Part print with two shaded views. Sizes in mm from the minimum x, y, z corner. A direction names the side the tool comes from. Round coordinates to 2 decimals unless told otherwise and drop trailing zeros. Write each loop counter-clockwise with the first axis right and the second up, starting at its lowest first coordinate (ties: lowest second). Pieces come first, ordered by that corner, then holes.
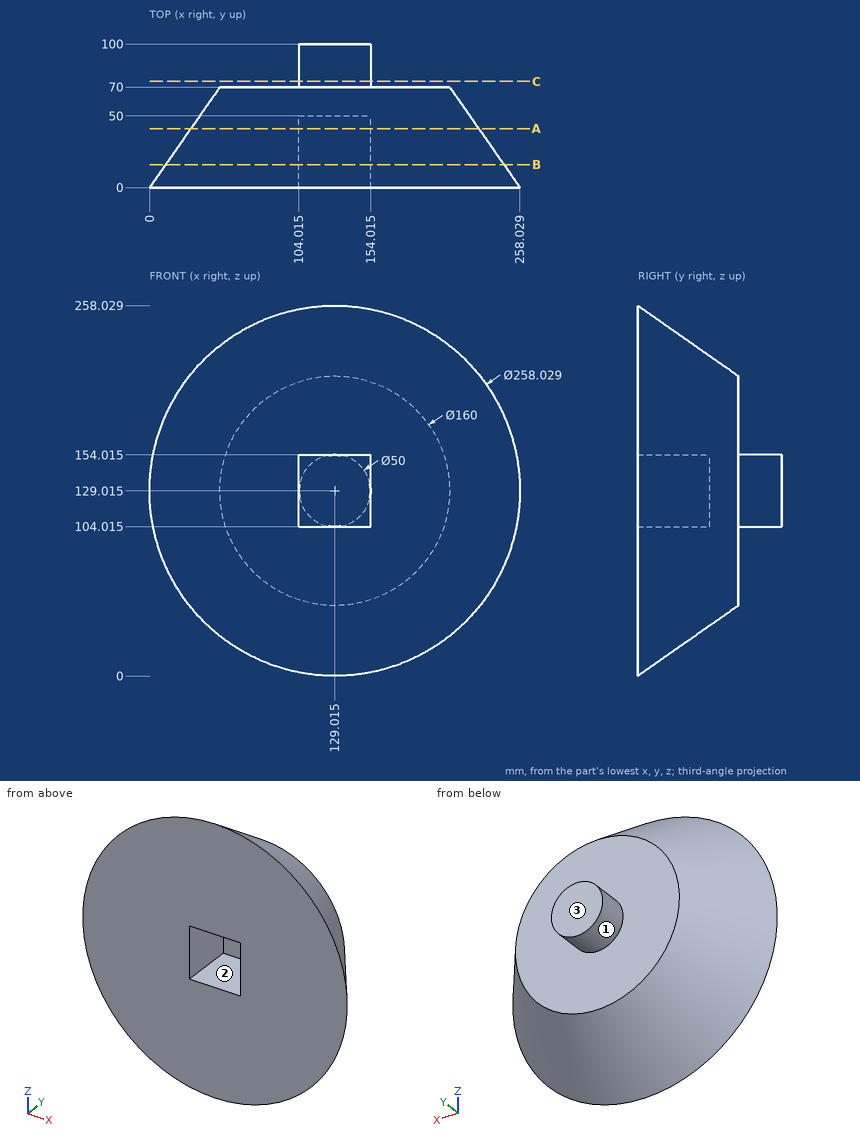
Q1. Cut at C-C on y = 74. Write the cut outline in (x, z) (1 decimal).
Values follow:
outline: circle Ø50 at (129, 129)
Q2. Cut at A-A on y = 41. Write the cut outline in (x, z) (1 decimal).
Values follow:
outline: circle Ø200.6 at (129, 129); hole (104, 104) - (154, 104) - (154, 154) - (104, 154) - close
Q3. Drop flat-ended pins along their axis: pin 1 (15 mm diameter, centred on x = 124.5, z = 134.5, fed in from -Y); pin 2 (10 mm diameter, centred on x = 219.5, z = 81.5, fed in from +Y) (1 decimal); pin 3 (6 mm diameter, centred on x = 72, y = 18, fed in from +Z). Give the stop position or say it passes through.
Values follow:
pin 1: stops at y = 50
pin 2: stops at y = 45.4
pin 3: stops at z = 233.41
Q4. Wall check: L1, parallel to Y at x = 71.5, z = 125.5; L2, parallel to Y at x = 232, z = 146.5 (1 decimal); L3, parallel to X at y = 12, z = 207 (1 decimal). Give the ranges that are in metal, low to high.
Values follow:
L1: y = 0 to 70
L2: y = 0 to 35.1
L3: x = 37 to 221
Q5. Which spindle directions (+Z, -Z, +X, -X, +Y, -Y) get a long thin tool onto all of the face, cutting with end or side? Do the marked faces 1, 2 and 3. Say none if no direction does.
Values follow:
face 1: +Y
face 2: -Y
face 3: +Z, -Z, +X, -X, +Y
Q6. Cut at B-B on y = 16. Write the cut outline in (x, z) (1 decimal).
Values follow:
outline: circle Ø235.6 at (129, 129); hole (104, 104) - (154, 104) - (154, 154) - (104, 154) - close
